For this review, take the finished solid that the model builds, in its own axes (mm). Give positions to 0.01 mm unless a question says otherwise; leave off trailing zeros. Loops run counter-clockwise (first coordinate to the right, second up) from the corner with the lowest first, then second, coordinate; pieces in that order, holes last. Notation, with made-up numbers: M 46,-15.5 L 86,-15.5 A31 cw 86,23.5 Z; hole C 49,-18 d3. An arc over 180 degrees is marked long. Use CSV: the item, a comma, the result in double quotes. Start each with the question number.
1. Insertion check: P1, Ø2.5, axis at x = 0, z = -8.5, coming from the -Y side; P2, Ø1, axis at x = -15, y = 3, coming from the -Z side. Each pin has a flat end and moves straight along its axis. Give the tip position at first contact, or say it passes through.
2. To check wall thickness, follow line 1 (X direction, y = 2.1, z = -12.5); line 2 (Z direction, x = -9.5, y = 0.9); line 3 (X direction, y = 3.2, z = 0). State the ranges of each line that lie inside material, in increasing order. Write a range as [from, to].
3. Take a section at A-A, the plane z = 12.5. Write out the cut boundary in (x, y).
4. Take a section at C-C, the plane x = 10. Write out the cut boundary in (y, z).
5. Take a section at B-B, the plane z = -8.5. Write out the cut boundary in (x, y), and give its area (3 significant figures).
6. Take a section at D-D, the plane y = 2.65. Write out the cut boundary in (x, z), and give its area (3 significant figures).
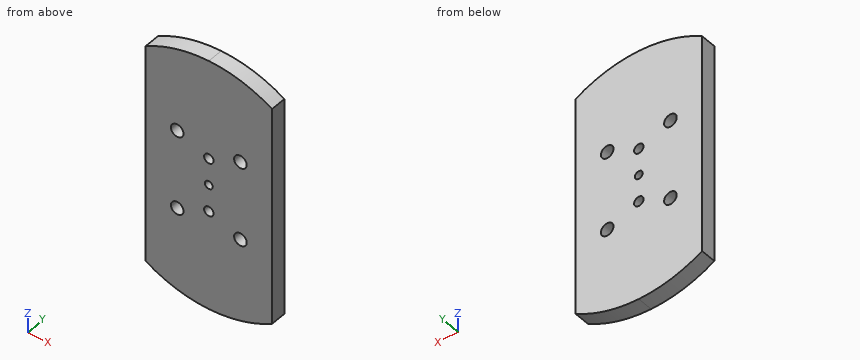
from build123d import *

# Parameters (mm, degrees)
ESQUISSE1_W               = 40
ESQUISSE1_H               = 80
BOSS_EXTRU_1_DEPTH        = 5
ESQUISSE2_R               = 1.5
ENL_V_MAT_EXTRU_1_DEPTH   = 5
ENL_V_START               = -5
ENL_V_MAT_EXTRU_5_DEPTH   = 5
ESQUISSE13_R              = 2
ENL_V_MAT_EXTRU_9_DEPTH   = 5
SYM_TRIE6_COPY_1_SKETCH_R = 2
SYM_TRIE6_COPY_1_DEPTH    = 5
ESQUISSE15_R              = 1.25
ENL_V_MAT_EXTRU_10_DEPTH  = 10


# Read off the part's stored shape, not the designer's step: Enlèv. mat.-Extru.5
with BuildPart() as part:
    # Esquisse1 → Boss.-Extru.1 (new body)
    with BuildSketch(Plane(origin=(0, 0, 0), x_dir=(1, 0, 0), z_dir=(0, 1, 0))):
        Rectangle(ESQUISSE1_W, ESQUISSE1_H)
    extrude(amount=BOSS_EXTRU_1_DEPTH)

    # Esquisse2 → Enlèv. mat.-Extru.1 (cut)
    with BuildSketch(Plane(origin=(0, 5, 0), x_dir=(1, 0, 0), z_dir=(0, 1, 0))):
        with Locations(Location((0, 8.5, 0), (0, 0, 270))):
            Circle(ESQUISSE2_R)
        with Locations(Location((0, -8.5, 0), (0, 0, 270))):
            Circle(ESQUISSE2_R)
    extrude(amount=-ENL_V_MAT_EXTRU_1_DEPTH, mode=Mode.SUBTRACT)

    # Enlèv. mat.-Extru.5 outline → Enlèv. mat.-Extru.5 (cut)
    with BuildSketch(Plane(origin=(0, 0, 0), x_dir=(-1, 0, 0), z_dir=(0, -1, 0)).offset(ENL_V_START)):
        with BuildLine():
            ThreePointArc((0, -40), (-10.352761804, -38.637033051), (-20, -34.641016151))
            Line((-20, -34.641016151), (-20, -40))
            Line((-20, -40), (0, -40))
        make_face()
        with BuildLine():
            ThreePointArc((20, -34.641016151), (10.352761804, -38.637033051), (0, -40))
            Line((0, -40), (20, -40))
            Line((20, -40), (20, -34.641016151))
        make_face()
        with BuildLine():
            Line((-20, 40), (-20, 34.641016151))
            ThreePointArc((-20, 34.641016151), (-10.352761804, 38.637033051), (0, 40))
            Line((0, 40), (-20, 40))
        make_face()
        with BuildLine():
            Line((20, 40), (0, 40))
            ThreePointArc((0, 40), (10.352761804, 38.637033051), (20, 34.641016151))
            Line((20, 34.641016151), (20, 40))
        make_face()
    extrude(amount=ENL_V_MAT_EXTRU_5_DEPTH, mode=Mode.SUBTRACT)

    # Esquisse13 → Enlèv. mat.-Extru.9 (cut)
    with BuildSketch(Plane(origin=(0, 5, 0), x_dir=(1, 0, 0), z_dir=(0, 1, 0))):
        with Locations(Location((-10, 12.5, 0), (0, 0, 270))):
            Circle(ESQUISSE13_R)
    enl_v_mat_extru_9 = extrude(amount=-ENL_V_MAT_EXTRU_9_DEPTH, mode=Mode.SUBTRACT)

    # Symétrie5: Enlèv. mat.-Extru.9 across plane
    add(enl_v_mat_extru_9.mirror(Plane(origin=(0, 0, 0), x_dir=(0, 0, 1), z_dir=(1, 0, 0))), mode=Mode.SUBTRACT)

    # Symétrie6: Enlèv. mat.-Extru.9 across plane
    add(enl_v_mat_extru_9.mirror(Plane.XY), mode=Mode.SUBTRACT)

    # Symétrie6 copy 1 sketch → Symétrie6 copy 1 (cut)
    with BuildSketch(Plane(origin=(0, 5, 0), x_dir=(-1, 0, 0), z_dir=(0, 1, 0))):
        with Locations(Location((-10, 12.5, 0), (0, 0, 270))):
            Circle(SYM_TRIE6_COPY_1_SKETCH_R)
    extrude(amount=-SYM_TRIE6_COPY_1_DEPTH, mode=Mode.SUBTRACT)

    # Esquisse15 → Enlèv. mat.-Extru.10 (cut)
    with BuildSketch(Plane(origin=(0, 5, 0), x_dir=(1, 0, 0), z_dir=(0, 1, 0))):
        with Locations(Location((0, 0, 0), (0, 0, 270))):
            Circle(ESQUISSE15_R)
    extrude(amount=-ENL_V_MAT_EXTRU_10_DEPTH, mode=Mode.SUBTRACT)


solid = part.part
Result set:
1,P1,"through"
1,P2,"z = -37.28"
2,line 1,"[-20, -12], [-8, 8], [12, 20]"
2,line 2,"[-38.86, -14.44], [-10.56, 10.56], [14.44, 38.86]"
2,line 3,"[-20, -1.25], [1.25, 20]"
3,outline,"M -20,0 L -12,0 L -12,5 L -20,5 Z; M -8,0 L 8,0 L 8,5 L -8,5 Z; M 12,0 L 20,0 L 20,5 L 12,5 Z"
4,outline,"M 0,-38.73 L 5,-38.73 L 5,-14.5 L 0,-14.5 Z; M 0,-10.5 L 5,-10.5 L 5,10.5 L 0,10.5 Z; M 0,14.5 L 5,14.5 L 5,38.73 L 0,38.73 Z"
5,outline,"M -20,0 L -1.5,0 L -1.5,5 L -20,5 Z; M 1.5,0 L 20,0 L 20,5 L 1.5,5 Z"
5,area,"185 mm2"
6,outline,"M -20,-34.64 A40 ccw 20,-34.64 L 20,34.64 A40 ccw -20,34.64 Z; hole C -10,-12.5 d4; hole C -10,12.5 d4; hole C 0,-8.5 d3; hole C 0,8.5 d3; hole C 0,0 d2.5; hole C 10,-12.5 d4; hole C 10,12.5 d4"
6,area,"2,990 mm2"
